from build123d import *

# Parameters (mm, degrees)
F0_W     = 99.4157642126
F0_H     = 52.1809085621
F1_DEPTH = 6.35
F4_D     = 4.064
F4_DEPTH = 12.7
F4_TIP   = 1.2209487779
F5_D     = 4.064
F5_DEPTH = 12.7
F5_TIP   = 1.2209487779
F6_W     = 13.2178254426
F6_H     = 4.296275205
F7_DEPTH = 25.4


with BuildPart() as f1:
    # F0 (on Front) → F1 (new body)
    with BuildSketch(Plane.XZ):
        with Locations((-0.4946067929, 26.4614112966)):
            Rectangle(F0_W, F0_H)
    extrude(amount=F1_DEPTH)

    # F4
    with Locations(Plane.YZ.offset(49.2132753134)):
        with Locations((-3.2103247941, 48.4527722001)):
            Hole(F4_D / 2, depth=F4_DEPTH)
            with Locations((0, 0, -(F4_DEPTH + F4_TIP / 2))):  # 118° drill point
                Cone(0, F4_D / 2, F4_TIP, mode=Mode.SUBTRACT)

    # F5
    with Locations(Plane(origin=(-50.2024888992, 0, 0), x_dir=(0, -1, 0), z_dir=(-1, 0, 0))):
        with Locations((3.1683039851, 48.47811535)):
            Hole(F5_D / 2, depth=F5_DEPTH)
            with Locations((0, 0, -(F5_DEPTH + F5_TIP / 2))):  # 118° drill point
                Cone(0, F5_D / 2, F5_TIP, mode=Mode.SUBTRACT)

    # F6 (on face) → F7 (cut)
    with BuildSketch(Plane(origin=(0, 0, 0.3709570155), x_dir=(1, 0, 0), z_dir=(0, 0, -1))):
        with Locations((0, 3.175)):
            Rectangle(F6_W, F6_H)
    extrude(amount=-F7_DEPTH, mode=Mode.SUBTRACT)


solid = f1.part
For this review, take the finished solid that the model builds, in its own axes (mm). A direction names the side the tool comes from. Give positions to 0.01 mm unless a question says otherwise; leave off trailing zeros. Loops run counter-clockwise (first coordinate to the right, second up) from the corner with the lowest first, then second, coordinate; pieces in that order, holes last. Notation, with made-up numbers: M -19.75,-30.75 L -8.75,-30.75 A36 ccw -8.75,6.25 Z; hole C 65,58.5 d7. An arc over 180 degrees is marked long. Answer as a JSON object with one key per item and string values. Group by question number.
Q1. Add section B-B on x = -3.5. Give the boundary of the cut face in (y, z).
Q2. Insertion check: P1, Ø3.5, axis at y = -3.17, z = 48.48, coming from the -X side; P2, Ø1.3, axis at x = -1.5, y = -2.5, coming from the -Z side. Each pin has a flat end and moves straight along its axis. Give the tip position at first contact, or say it passes through.
Q3. Add section A-A on z = 21.5. Give the boundary of the cut face in (x, y), and give its area (3 significant figures).
Q4. For probe 1 along X at (y, z) = (-2.25, 22.5); probe 2 along Y at (x, z) = (3, 22), list the stretches that pass through material, from the lowest coordinate up. Write a range as [from, to].
Q5. Mouldability with a two-part tool opening along Y and no side actions: class faces 4 (the conical face through (-36.494, -3.092, 48.134)), 5 (the flat face through (-1, 0, 27)), 6 (the cylindrical face through (42.77, -5.15, 49.06)), 7 (the flat face through (49.213, -3, 26)) as +Y half, -Y half, draft (parallel to the pull), parting line (faces both ways), or undercut.
Q6. Tool access review of faces 1 (the flat face through (0, -1.027, 13)), 2 (the flat face through (-50.202, -3, 26)), 3 (the cylindrical face through (-43.764, -2.231, 46.675)): name each direction out of +Z, -Z, +X, -X, +Y, -Y from which nothing blocks a thin tool from reaching the whole face with its end or side.
Checked values:
{
 "1": {"outline": "M -6.35,0.37 L -5.32,0.37 L -5.32,25.77 L -1.03,25.77 L -1.03,0.37 L 0,0.37 L 0,52.55 L -6.35,52.55 Z"},
 "2": {"P1": "x = -37.33", "P2": "z = 25.77"},
 "3": {"outline": "M -50.2,-6.35 L 49.21,-6.35 L 49.21,0 L -50.2,0 Z; hole M -6.61,-5.32 L 6.61,-5.32 L 6.61,-1.03 L -6.61,-1.03 Z", "area": "575 mm²"},
 "4": {"probe 1": "[-50.2, -6.61], [6.61, 49.21]", "probe 2": "[-6.35, -5.32], [-1.03, 0]"},
 "5": {"face 4": "undercut", "face 5": "+Y half", "face 6": "undercut", "face 7": "draft"},
 "6": {"face 1": "-Z", "face 2": "+Z, -Z, -X, +Y, -Y", "face 3": "-X"}
}
